Could you check a few things on this model? Use its own coordinates, in mm. A direction names the side the tool comes from. Give positions to 0.01 mm unless a question says otherwise; leave off trailing zeros. Order: outer loops, then holes, each group sorted by start corner. A loop starts at its lowest first (then second) coordinate and runs counter-clockwise, first axis right, second up. Notation, with made-up numbers: M 27,-8.5 L 59,-8.5 A23 cw 59,7.5 Z; hole C -33,38.5 d6. An arc over 180 degrees is marked long. Return JSON: item names as keys, results as strings. Group by question number.
```python
from build123d import *

# Parameters (mm, degrees)
F0_W     = 36
F0_H     = 68
F1_DEPTH = 750
F3_DEPTH = 36
F5_DEPTH = 18


with BuildPart() as f1:
    # F0 (on Front) → F1 (new body)
    with BuildSketch(Plane.XZ):
        Rectangle(F0_W, F0_H)
    extrude(amount=F1_DEPTH)

    # F2 (on face) → F3 (cut, through all)
    with BuildSketch(Plane(origin=(-18, 0, 0), x_dir=(0, -1, 0), z_dir=(-1, 0, 0))):
        Polygon((18.220545, -34), (0, 34), (0, -34), align=None)
        Polygon((750, 34), (670, 34), (688.220545, -34), (750, -34), align=None)
    extrude(amount=-F3_DEPTH, mode=Mode.SUBTRACT)

    # F4 (on face) → F5 (cut)
    with BuildSketch(Plane(origin=(-18, 0, 0), x_dir=(0, -1, 0), z_dir=(-1, 0, 0))):
        Polygon((670, 34), (599.5, 34), (617.720545, -34), (688.220545, -34), align=None)
    extrude(amount=-F5_DEPTH, mode=Mode.SUBTRACT)


solid = f1.part
```
1. If we mould it in two halves opening along Y, with no side actions, what happens to faces 1 (the flat face through (8.87, -678.98, 0.48)), 2 (the flat face through (0, -330, 34)), 3 (the flat face through (-0.25, -9.24, -0.48))? For each: pulls with the +Y half, pulls with the -Y half, needs draft (parallel to the pull), parting line crosses it, or undercut.
2. Imagine slicing it at A-A, the plane x = 11.5. Please give me the cut outline in (y, z).
3. I need wall thicknesses on L1, parallel to X at y = -639, z = -14; L2, parallel to Y at x = 10, z = 24.5; L3, parallel to Y at x = 13, z = -21. Which ranges of each line are inside material? Lowest first, please. Write a range as from..to.
4. For pin 1 (6 mm diameter, centred on x = -13, z = 19.5, fed in from -Y); pin 2 (1.5 mm diameter, centred on x = -1, z = 11.5, fed in from +Y); pin 3 (1.5 mm diameter, centred on x = -12.5, z = -12, fed in from +Y), each with a flat end and sliding along its axis, tell me the tip position at first contact or that it passes through.
5. Imagine slicing it at B-B, the plane z = -13.5. Please give me the cut outline in (x, y), plus the area to 3 significant figures.
6. Which directions (+Z, -Z, +X, -X, +Y, -Y) give clear straight access to the entire face, cutting with the end or side of a thin tool? Please do faces 4 (the flat face through (18, -339, 0)), 5 (the flat face through (0, -643, 0)).
Values:
{
 "1": {"face 1": "pulls with the -Y half", "face 2": "needs draft", "face 3": "pulls with the +Y half"},
 "2": {"outline": "M -688.22,-34 L -18.22,-34 L 0,34 L -670,34 Z"},
 "3": {"L1": "x = 0..18", "L2": "y = -672.55..-2.55", "L3": "y = -684.74..-14.74"},
 "4": {"pin 1": "stops at y = -604.19", "pin 2": "stops at y = -5.83", "pin 3": "stops at y = -12.12"},
 "5": {"outline": "M -18,-612.23 L 0,-612.23 L 0,-682.73 L 18,-682.73 L 18,-12.73 L -18,-12.73 Z", "area": "22,900 mm²"},
 "6": {"face 4": "+Z, -Z, +X, +Y, -Y", "face 5": "+Z, -X, -Y"}
}
